Read the model definition and answer for the solid it produces. Units are mm, in the model's axes. Face numbers are marked on the shaded views. Give positions to 0.01 mm unless a question says otherwise; leave off trailing zeros. Write each loop counter-clockwise with the first axis right and the second up, starting at its lowest first coordinate (ties: lowest second). Pieces come first, ordered by that corner, then holes. Notation, with made-up numbers: (-39, 69) - (5, 69) arc R13 ccw to (5, 79) - close; hole circle Ø9 at (-12.75, 41.25). An arc over 180 degrees is marked (long way). Answer as a JSON object with one key per item and string values. Group by question number.
```python
from build123d import *

# Parameters (mm, degrees)
FILLET1_R       = 0.2
FILLET2_R       = 0.25
HEX_2_DEPTH     = 2.5
THDSCHPAT_COUNT = 29
THDSCHPAT_PITCH = 0.785714286


with BuildPart() as part:
    # BodySke → Base-Revolve (revolve)
    with BuildSketch(Plane.XY):
        Polygon((0, 0), (0, 4.25), (5, 4.25), (5, 2.5), (44.555, 2.5), (45, 2.055), (45, 0), align=None)
    revolve(axis=Axis((-31.75, 0, 0), (1, 0, 0)))

    # Fillet1
    fillet1_edges = [part.edges().sort_by_distance(p)[0] for p in [
        (5, -2.5, 0),
    ]]
    fillet(fillet1_edges, radius=FILLET1_R)

    # Fillet2
    fillet2_edges = [part.edges().sort_by_distance(p)[0] for p in [
        (0, -4.25, 0),
    ]]
    fillet(fillet2_edges, radius=FILLET2_R)

    # Sketch2 → Hex-PreBroach (revolve, cut)
    with BuildSketch(Plane.XY):
        Polygon((0, 2.042), (2.5, 2.042), (3.67894925, 0), (0, 0), align=None)
    revolve(axis=Axis((0, 0, 0), (1, 0, 0)), mode=Mode.SUBTRACT)

    # Sketch3 → Hex 2 (cut)
    with BuildSketch(Plane(origin=(0, 0, 0), x_dir=(0, 0.5, 0.866025404), z_dir=(-1, 0, 0))):
        Polygon((1.17894925, 2.042), (-1.17894925, 2.042), (-2.357898499, 0), (-1.17894925, -2.042), (1.17894925, -2.042), (2.357898499, 0), align=None)
    extrude(amount=-HEX_2_DEPTH, mode=Mode.SUBTRACT)

    # ThdSchSke → ThreadSchematic (revolve, cut)
    with BuildSketch(Plane.XY):
        Polygon((23, -2.055), (22.688407645, -2.5), (22.688407645, -3.125), (23.311592355, -3.125), (23.311592355, -2.5), align=None)
    threadschematic = revolve(axis=Axis((-3.175, 0, 0), (1, 0, 0)), mode=Mode.SUBTRACT)

    # ThdSchPat: ThreadSchematic ×29
    with Locations(*[(i * THDSCHPAT_PITCH, 0, 0) for i in range(1, THDSCHPAT_COUNT)]):
        add(threadschematic, mode=Mode.SUBTRACT)


solid = part.part
```
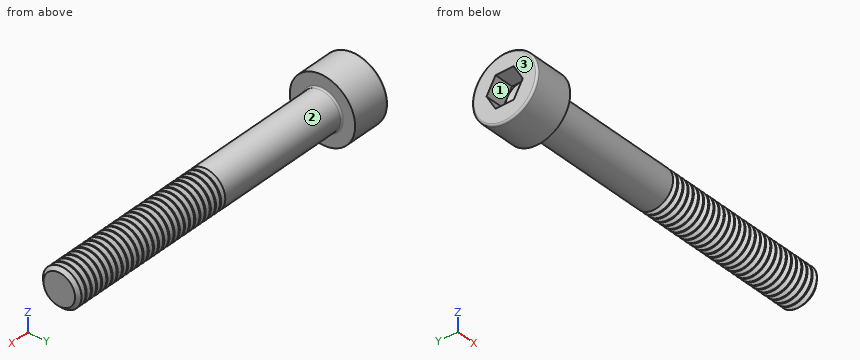
1) Find the intervals of material crossed by line 1 (X direction, y = 2, z = -3); line 2 (Y direction, x = 10, z = 0); line 3 (Y direction, x = 19, z = 0.75), in increasing order. Write a range as [from, to].
2) For a pull along Y with two mould halves and no side action, classify the marked faces 1, 2 and 3 as released by +Y, released by -Y, zero draft, split by the parting line, or undercut.
3) Find section A-A, the plane x = 12.5. Write down the section's boundary in (y, z).
4) Flat-ended cylindrical pins translate along their axes: pin 1 Ø4 at (x, y) = (24, -1.5) entering from +Z; pin 2 Ø1.5 at (x, z) = (36, 2.5) entering from +Y; pin 3 Ø0.5 at (y, z) = (2, 0) entering from -X. Find the tip coordinate at first contact, or state that the pin passes through.
Values follow:
{
 "1": {"line 1": "x = [0, 5]", "line 2": "y = [-2.5, 2.5]", "line 3": "y = [-2.38, 2.38]"},
 "2": {"face 1": "undercut", "face 2": "split by the parting line", "face 3": "zero draft"},
 "3": {"outline": "circle Ø5 at (0, 0)"},
 "4": {"pin 1": "stops at z = 2.5", "pin 2": "stops at y = 1.79", "pin 3": "stops at x = 2.5"}
}
